Check sheet for the modelled part. Datum: model origin and axes. Units: mm. A direction names the side the tool comes from. Round coordinates to 2 decimals unless told otherwise and drop trailing zeros.
Item 1: Tool access check on faces 1 (the flat face through (89.824, -6, -4)), 2 (the flat face through (-3, -6, 50.8)). Record the directions out of +Z, -Z, +X, -X, +Y, -Y that give a thin tool (end or side, any length) a straight path to the whole face; none if there is none.
Item 2: Material ranges on line 1 (X direction, y = -6.35, z = 47.25); line 2 (X direction, y = -1.5, z = 41.5); line 3 (Z direction, x = -107, y = -7), recorded low to high.
Item 3: Go/stop test with flat-tipped pins: pin 1 Ø6.5 at (y, z) = (-8.5, -31) entering from -X; pin 2 Ø4 at (y, z) = (-5.5, -22.5) entering from +X; pin 3 Ø2 at (x, z) = (-28, 1.5) entering from -Y. Record where each tip stops, or that it passes through.
Item 4: Release check for a two-part mould opening along X. For faces 3 (the flat face through (190.5, -6, -45)), 4 (the cylindrical face through (-179.57, -6.49, -44.54)), 5 (the flat face through (-190.5, -6, -45)) record: +X half, -X half, draft (parallel to the pull), parting line (faces both ways), or undercut.
from build123d import *

# Parameters (mm, degrees)
F0_W     = 381
F0_H     = 101.6
F1_DEPTH = 12.7
F2_W     = 44.543445
F2_H     = 28.842324
F2_W_2   = 27.413249
F2_H_2   = 9.482801
F2_W_3   = 39.025373
F2_H_3   = 11.841384
F2_W_4   = 67.109051
F2_H_4   = 27.095137
F2_W_5   = 66.744328
F2_H_5   = 14.588922
F2_W_6   = 18.965602
F2_W_7   = 37.566483
F2_H_6   = 8.023907
F2_W_8   = 42.672605
F2_H_7   = 14.588925
F2_W_9   = 17.506707
F2_H_8   = 13.468034
F2_W_10  = 8.568198
F2_H_9   = 12.874041
F2_W_11  = 21.838954
F2_H_10  = 13.367074
F2_W_12  = 14.083162
F2_H_11  = 21.530468
F2_W_13  = 19.033331
F2_H_12  = 14.701502
F2_W_14  = 66.379599
F2_H_13  = 4.741401
F2_W_15  = 58.355704
F2_H_14  = 26.989511
F2_W_16  = 25.165893
F2_H_15  = 4.376677
F2_W_17  = 30.636735
F2_H_16  = 10.46557
F2_W_18  = 52.520126
F2_H_17  = 8.157725
F2_W_19  = 33.919238
F2_H_18  = 7.933862
F2_W_20  = 14.953643
F2_H_19  = 13.494756
F2_W_21  = 24.07172
F2_H_20  = 15.053647
F2_W_22  = 21.153938
F2_H_21  = 14.091857
F2_W_23  = 47.352944
F2_H_22  = 76.2
F2_W_24  = 24.159947
F2_H_23  = 12.841732
F2_W_25  = 29.462242
F3_DEPTH = 12.701
F4_R     = 3.175
F5_DEPTH = 101.601
F6_R     = 1.5875
F7_DEPTH = 12.701


with BuildPart() as f1:
    # F0 (on Front) → F1 (new body)
    with BuildSketch(Plane.XZ):
        Rectangle(F0_W, F0_H)
    extrude(amount=F1_DEPTH)

    # F2 (on face) → F3 (cut, through all)
    with BuildSketch(Plane.XZ.offset(12.7)):
        with Locations((-103.138441, 31.688611)):
            Rectangle(F2_W, F2_H)
        with Locations((-139.799008, 2.707727)):
            Rectangle(F2_W_2, F2_H_2)
        with Locations((-110.591656, -36.794207)):
            Rectangle(F2_W_3, F2_H_3)
        with Locations((-16.675455, -10.475118)):
            Rectangle(F2_W_4, F2_H_4)
        with Locations((8.308077, 38.085867)):
            Rectangle(F2_W_5, F2_H_5)
        with Locations((-74.301707, 4.166619)):
            Rectangle(F2_W_6, F2_H_2)
        with Locations((-86.519928, -20.634552)):
            Rectangle(F2_W_7, F2_H_6)
        with Locations((-9.928079, -40.694322)):
            Rectangle(F2_W_8, F2_H_7)
        with Locations((-58.983334, -37.607532)):
            Rectangle(F2_W_9, F2_H_8)
        with Locations((-142.047623, -39.836879)):
            Rectangle(F2_W_10, F2_H_9)
        with Locations((-143.57688, -18.692414)):
            Rectangle(F2_W_11, F2_H_10)
        with Locations((-143.858196, 33.532733)):
            Rectangle(F2_W_12, F2_H_11)
        with Locations((-47.710783, 16.634559)):
            Rectangle(F2_W_13, F2_H_12)
        with Locations((96.753428, 13.467059)):
            Rectangle(F2_W_14, F2_H_13)
        with Locations((99.306492, -29.387906)):
            Rectangle(F2_W_15, F2_H_14)
        with Locations((49.886511, -23.91706)):
            Rectangle(F2_W_16, F2_H_15)
        with Locations((100.765379, 38.81371)):
            Rectangle(F2_W_17, F2_H_16)
        with Locations((92.741473, 25.373465)):
            Rectangle(F2_W_18, F2_H_17)
        with Locations((106.78331, -3.966931)):
            Rectangle(F2_W_19, F2_H_18)
        with Locations((42.227322, -9.87522)):
            Rectangle(F2_W_20, F2_H_19)
        with Locations((20.161576, 16.649821)):
            Rectangle(F2_W_21, F2_H_20)
        with Locations((-55.700827, 36.834504)):
            Rectangle(F2_W_22, F2_H_21)
        with Locations((166.823528, 0)):
            Rectangle(F2_W_23, F2_H_22)
        with Locations((41.271404, -39.226733)):
            Rectangle(F2_W_24, F2_H_23)
        with Locations((-175.768879, 0)):
            Rectangle(F2_W_25, F2_H_22)
    extrude(amount=-F3_DEPTH, mode=Mode.SUBTRACT)

    # F4 (on face) → F5 (cut, through all)
    with BuildSketch(Plane(origin=(0, 0, -50.8), x_dir=(1, 0, 0), z_dir=(0, 0, -1))):
        with Locations((166.722789, 5.933621)):
            Circle(F4_R)
        with Locations((-176.396297, 6.35)):
            Circle(F4_R)
    extrude(amount=-F5_DEPTH, mode=Mode.SUBTRACT)

    # F6 (on face) → F7 (cut, through all)
    with BuildSketch(Plane.XZ.offset(12.7)):
        with Locations((-119.230784, -1.5875)):
            Circle(F6_R)
        with Locations((133.051559, 0)):
            Circle(F6_R)
    extrude(amount=-F7_DEPTH, mode=Mode.SUBTRACT)


solid = f1.part
Response values:
1. face 1: +Y, -Y
1. face 2: +Z, +X, -X, +Y, -Y
2. line 1: x = -190.5 to -179.57, -173.22 to 163.58, 169.87 to 190.5
2. line 2: x = -190.5 to -150.9, -136.82 to -125.41, -80.87 to -66.28, -45.12 to -25.06, 41.68 to 85.45, 116.08 to 190.5
2. line 3: z = -50.8 to -42.71, -30.87 to 17.27, 46.11 to 50.8
3. pin 1: stops at x = -161.04
3. pin 2: stops at x = 143.15
3. pin 3: passes through
4. face 3: +X half
4. face 4: undercut
4. face 5: -X half
